```python
from build123d import *

# Parameters (mm, degrees)
SKETCH2_R          = 1.65
CUT_EXTRUDE1_DEPTH = 12.5


with BuildPart() as part:
    # Sketch1 → Revolve1 (revolve)
    with BuildSketch(Plane.XY, mode=Mode.PRIVATE) as revolve1_sk:
        with BuildLine():
            Line((0, 4.5), (0, -4.5))
            Line((0, -4.5), (3.5, -4.5))
            Line((3.5, -4.5), (3.5, -3.5))
            Line((3.5, -3.5), (2, -2))
            Line((2, -2), (2, -0.7))
            ThreePointArc((2, -0.7), (2.9, 1.4), (2, 3.5))
            Line((2, 3.5), (2, 4.5))
            Line((2, 4.5), (0, 4.5))
        make_face()
    revolve(revolve1_sk.sketch.rotate(Axis((0, 9.816629846, 0), (0, -1, 0)), 90), axis=Axis((0, 9.816629846, 0), (0, -1, 0)))

    # Sketch2 → Cut-Extrude1 (cut)
    with BuildSketch(Plane(origin=(0, 4.5, 0), x_dir=(1, 0, 0), z_dir=(0, 1, 0))):
        with Locations(Location((0, 0, 0), (0, 0, 270))):
            Circle(SKETCH2_R)
    extrude(amount=-CUT_EXTRUDE1_DEPTH, mode=Mode.SUBTRACT)


solid = part.part
```
The listing builds one solid part. Answer for the finished solid, in the listing's coordinates (mm). A direction names the side the tool comes from. Round coordinates to 2 decimals unless told otherwise and drop trailing zeros. Loops run counter-clockwise (first coordinate to the right, second up) from the corner with the lowest first, then second, coordinate; pieces in that order, holes last.
1) Consider line 1 (X direction, y = -1.5, z = 0); line 2 (Z direction, x = 0.25, y = 2.5); line 3 (Z direction, x = -1, y = 0.5). Determine where each line is inside the solid, lowest interval first.
Outcome:
line 1: x = -2 to -1.65, 1.65 to 2
line 2: z = -2.67 to -1.63, 1.63 to 2.67
line 3: z = -2.57 to -1.31, 1.31 to 2.57
2) A cutting plane is placed at D-D on y = -1. Determine the outline of the cut face in (x, z).
Outcome:
outline: circle Ø4 at (0, 0); hole circle Ø3.3 at (0, 0)
3) A cutting plane is placed at A-A on x = 0. Determine the outline of the cut face in (y, z).
Outcome:
outline: (-4.5, -3.5) - (-3.5, -3.5) - (-2, -2) - (-0.7, -2) arc R2.9 ccw to (3.5, -2) - (4.5, -2) - (4.5, -1.65) - (-4.5, -1.65) - close; (-4.5, 1.65) - (4.5, 1.65) - (4.5, 2) - (3.5, 2) arc R2.9 ccw to (-0.7, 2) - (-2, 2) - (-3.5, 3.5) - (-4.5, 3.5) - close
4) A cutting plane is placed at C-C on y = -2.75. Determine the outline of the cut face in (x, z).
Outcome:
outline: circle Ø5.5 at (0, 0); hole circle Ø3.3 at (0, 0)
5) For faces 4 (the face through (2, -1, 0)), 5 (the face through (3.105, -3.993, 1.615)), determine the directions among +Z, -Z, +X, -X, +Y, -Y from which every point of the face is accessible in a straight line to the end or side of a thin tool.
Outcome:
face 4: none
face 5: +Y, -Y
6) A cutting plane is placed at B-B on z = 0. Determine the outline of the cut face in (x, y).
Outcome:
outline: (-3.5, -4.5) - (-1.65, -4.5) - (-1.65, 4.5) - (-2, 4.5) - (-2, 3.5) arc R2.9 ccw to (-2, -0.7) - (-2, -2) - (-3.5, -3.5) - close; (1.65, -4.5) - (3.5, -4.5) - (3.5, -3.5) - (2, -2) - (2, -0.7) arc R2.9 ccw to (2, 3.5) - (2, 4.5) - (1.65, 4.5) - close
7) For a pull along Z with two mould halves and no side action, classify faces 1 (the face through (-1, 0.06, -1.31)), 2 (the face through (2, -4.5, -1)), 3 (the face through (2, 4, 0)) as released by +Z, released by -Z, zero draft, split by the parting line, or undercut.
Outcome:
face 1: undercut
face 2: zero draft
face 3: split by the parting line
8) Given P1, Ø4, axis at x = 2, z = 1, coming from the +Y side; P2, Ø2, axis at x = 2, y = -3, coming from the +Z side; P3, Ø4, axis at y = -1.5, z = 2, coming from the +X side; P4, Ø4, axis at y = -0.5, z = 1.5, coming from the +X side, each flat-ended and moving along its own axis, determine where each tip first touches the part or whether it passes through.
Outcome:
P1: stops at y = 4.5
P2: stops at z = 3.31
P3: stops at x = 3.11
P4: stops at x = 2.87
